Build history of the part. All positions in model axes, mm. Face numbers are marked on the shaded views. A direction names the side the tool comes from. Give positions to 0.01 mm unless a question says otherwise; leave off trailing zeros. Order: outer loops, then holes, each group sorted by start corner. A loop starts at its lowest first (then second) coordinate and runs counter-clockwise, first axis right, second up. Notation, with made-up numbers: M -35.5,-15.75 L -23.5,-15.75 A22 ccw -23.5,15.25 Z; hole C 69.25,54 d8. An arc over 180 degrees is marked long. Answer as CSV lines item,"result".
from build123d import *

# Parameters (mm, degrees)
SKETCH1_R           = 4.5
BOSS_EXTRUDE1_DEPTH = 8
BOSS_EXTRUDE1_DRAFT = -3.5
BOSS_EXTRUDE2_DEPTH = 8
SKETCH3_R           = 6
BOSS_EXTRUDE3_DEPTH = 2
SKETCH9_R           = 4.5
BOSS_EXTRUDE6_DEPTH = 0.5
FILLET1_R           = 1.9
SKETCH4_R           = 3.75
BOSS_EXTRUDE4_DEPTH = 1
SKETCH5_R           = 6
BOSS_EXTRUDE5_DEPTH = 1
SKETCH6_R           = 3
CUT_EXTRUDE1_DEPTH  = 8.5
CUT_EXTRUDE2_DEPTH  = 8
SKETCH8_R           = 3.175
CUT_EXTRUDE3_DEPTH  = 4


with BuildPart() as part:
    # Sketch1 → Boss-Extrude1 (with draft: the straight prism first)
    with BuildSketch(Plane.XY):
        Circle(SKETCH1_R)
    extrude(amount=BOSS_EXTRUDE1_DEPTH)
    # Boss-Extrude1: the draft: its side faces are tilted about the plane it starts from
    boss_extrude1_sides = [part.faces().sort_by_distance(p)[0] for p in [
        (-4.5, 0, 4),
    ]]
    draft(boss_extrude1_sides, Plane.XY, BOSS_EXTRUDE1_DRAFT)

    # Sketch2 → Boss-Extrude2 (add)
    with BuildSketch(Plane.XY.offset(8)):
        Polygon((6.92820323, 0), (3.464101615, 6), (-3.464101615, 6), (-6.92820323, 0), (-3.464101615, -6), (3.464101615, -6), align=None)
    extrude(amount=BOSS_EXTRUDE2_DEPTH)

    # Sketch3 → Boss-Extrude3 (add)
    with BuildSketch(Plane.XY.offset(16)):
        with Locations(Location((0, 0, 0), (0, 0, 150))):
            Circle(SKETCH3_R)
    extrude(amount=BOSS_EXTRUDE3_DEPTH)

    # Sketch9 → Boss-Extrude6 (add)
    with BuildSketch(Plane.XY.offset(18)):
        Circle(SKETCH9_R)
    extrude(amount=BOSS_EXTRUDE6_DEPTH)

    # Fillet1
    # the kernel refuses this fillet: 1.9 mm, written as the material it takes off along each edge
    with BuildSketch(Plane(origin=(0, 0, 18), x_dir=(-0.8660254037844387, 0.49999999999999994, 0), z_dir=(0.49999999999999994, 0.8660254037844387, 0))) as fillet1_piece_1:
        with BuildLine():
            CenterArc((4.1, -1.857417562), FILLET1_R, 0, 77.846802531)
            Line((4.5, 0), (4.508, 0.037148351))
            ThreePointArc((4.508, 0.037148351), (5.25, 0.038), (6, 0.038))
            Line((6, 0.038), (6.038, 0))
            Line((6.038, 0), (6.038, -1.857417562))
            Line((6.038, -1.857417562), (6, -1.857417562))
        make_face()
    revolve(axis=Axis((0, 0, 18), (0, 0, 1)), mode=Mode.SUBTRACT)

    # Sketch4 → Boss-Extrude4 (add)
    with BuildSketch(Plane.XY.offset(18.5)):
        Circle(SKETCH4_R)
    extrude(amount=BOSS_EXTRUDE4_DEPTH)

    # Sketch5 → Boss-Extrude5 (add)
    with BuildSketch(Plane.XY.offset(19.5)):
        with Locations(Location((0, 0, 0), (0, 0, 150))):
            Circle(SKETCH5_R)
    extrude(amount=BOSS_EXTRUDE5_DEPTH)

    # Sketch6 → Cut-Extrude1 (cut)
    with BuildSketch(Plane.XY.offset(20.5)):
        Circle(SKETCH6_R)
    extrude(amount=-CUT_EXTRUDE1_DEPTH, mode=Mode.SUBTRACT)

    # Sketch7 → Cut-Extrude2 (cut)
    with BuildSketch(Plane.XY.offset(12)):
        Polygon((0, -2.309401077), (2, -1.154700538), (2, 1.154700538), (0, 2.309401077), (-2, 1.154700538), (-2, -1.154700538), align=None)
    extrude(amount=-CUT_EXTRUDE2_DEPTH, mode=Mode.SUBTRACT)

    # Sketch8 → Cut-Extrude3 (cut)
    with BuildSketch(Plane(origin=(0, 0, 0), x_dir=(-1, 0, 0), z_dir=(0, 0, -1))):
        Circle(SKETCH8_R)
    extrude(amount=-CUT_EXTRUDE3_DEPTH, mode=Mode.SUBTRACT)


solid = part.part
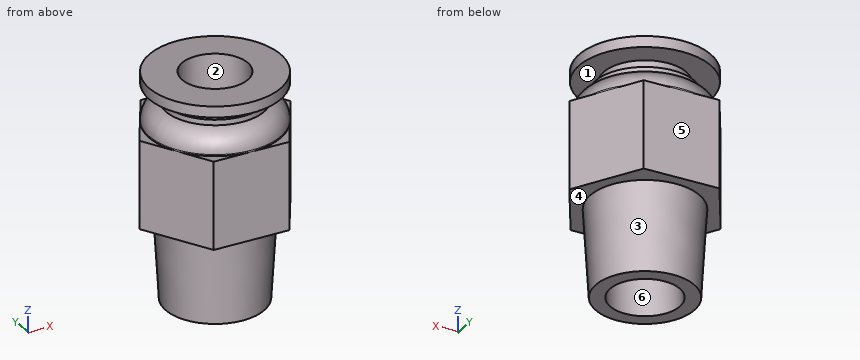
Item 1: Band-saw the part on D-D (z = 2). Give the cut face in (x, y) (3 decimals).
Geometry says:
outline,"C 0,0 d9.245; hole C 0,0 d6.35"
Item 2: Probe line 1 along Y through (x, z) = (0, 15.5); line 2 along Z through (x, y) = (1, -4); line 3 along Z through (x, y) = (-1.5, 1.5). List the from-to ranges inside material, lowest first. Write a range as from..to.
Geometry says:
line 1,"y = -6..-3, 3..6"
line 2,"z = 0..18.5, 19.5..20.5"
line 3,"z = 4..12"
Item 3: Band-saw the part on C-C (z = 17.25). Give the cut face in (x, y).
Geometry says:
outline,"C 0,0 d11.29; hole C 0,0 d6"
Item 4: Band-saw the part on A-A (z = 14.5). Give the cut face in (x, y).
Geometry says:
outline,"M -6.93,0 L -3.46,-6 L 3.46,-6 L 6.93,0 L 3.46,6 L -3.46,6 Z; hole C 0,0 d6"
Item 5: Band-saw the part on B-B (z = 11.75). Give the cut face in (x, y), and give its area (3 significant figures).
Geometry says:
outline,"M -6.93,0 L -3.46,-6 L 3.46,-6 L 6.93,0 L 3.46,6 L -3.46,6 Z; hole M -2,-1.15 L 0,-2.31 L 2,-1.15 L 2,1.15 L 0,2.31 L -2,1.15 Z"
area,"111 mm2"
Item 6: Drop flat-ended pins along their axis: pin 1 (3 mm diameter, centred on x = -1, y = 0, fed in from -Z); pin 2 (3 mm diameter, centred on y = 2.5, z = 8.5, fed in from +X); pin 3 (2 mm diameter, centred on x = 4.5, z = 3.5, fed in from -Y). Give the stop position or say it passes through.
Geometry says:
pin 1,"stops at z = 4"
pin 2,"stops at x = 6.35"
pin 3,"stops at y = -3.16"
Item 7: 3-axis set-ups, long thin cutter, end or side, ignore diameter. For the marked faces 1, 2 and 3: which of +Z, -Z, +X, -X, +Y, -Y reach the whole face in a straight line?
Geometry says:
face 1,"none"
face 2,"+Z"
face 3,"-Z"
Item 8: Pull direction Y, two halves, no side cores. Call the marked faces 4, 5 and 6: released by +Y, released by -Y, zero draft, split by the parting line, or undercut.
Geometry says:
face 4,"zero draft"
face 5,"released by +Y"
face 6,"undercut"
